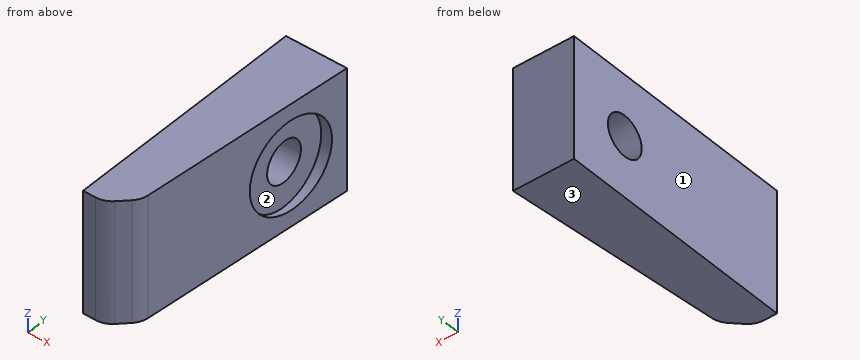
from build123d import *

# Parameters (mm, degrees)
EXTRUDE_1_DEPTH     = 30
SKETCH_3_R          = 5
CUT_EXTRUDE_2_DEPTH = 21
CUT_EXTRUDE_START   = -15
SKETCH_5_R          = 11
CUT_EXTRUDE_3_DEPTH = 3


with BuildPart() as part:
    # Эскиз1 → Бобышка-Вытянуть1 (new body)
    with BuildSketch(Plane.XY):
        with BuildLine():
            Line((0, 0), (0, -60))
            Line((0, -60), (3.117055694, -60))
            ThreePointArc((3.117055694, -60), (5.030472856, -59.619397663), (6.6525896, -58.535533906))
            Line((6.6525896, -58.535533906), (8.901294402, -56.286829104))
            ThreePointArc((8.901294402, -56.286829104), (9.897299431, -54.864386507), (10.346733987, -53.187073912))
            Line((10.346733987, -53.187073912), (15, 0))
            Line((15, 0), (0, 0))
        make_face()
    extrude(amount=EXTRUDE_1_DEPTH)

    # Эскиз3 → Вырез-Вытянуть2 (cut)
    with BuildSketch(Plane.ZY):
        with Locations((15, -15)):
            Circle(SKETCH_3_R)
    extrude(amount=-CUT_EXTRUDE_2_DEPTH, mode=Mode.SUBTRACT)

    # Эскиз5 → Вырез-Вытянуть3 (cut)
    with BuildSketch(Plane.ZY.offset(CUT_EXTRUDE_START)):
        with Locations((15, -15)):
            Circle(SKETCH_5_R)
    extrude(amount=CUT_EXTRUDE_3_DEPTH, mode=Mode.SUBTRACT)


solid = part.part
Can you work these out from the model? Positions are in its coordinate system, mm. Face numbers are marked on the shaded views. Give positions to 0.01 mm unless a question says otherwise; leave off trailing zeros. Loops run counter-clockwise (first coordinate to the right, second up) from the corner with the lowest first, then second, coordinate; pieces in that order, holes last. Notation, with made-up numbers: (32.25, 2) - (50.25, 2) arc R12 ccw to (50.25, 19) - close; hole circle Ø5 at (-14.75, -20). An arc over 180 degrees is marked (long way). One line per item, written item: value.
(1) If we section it at D-D, the plane x = 4: List the corners of the cut face in (y, z) for me.
Verdict:
outline: (-59.92, 0) - (0, 0) - (0, 30) - (-59.92, 30) - close; hole circle Ø10 at (-15, 15)
(2) If we section it at C-C, the plane z = 27.75: List the corners of the cut face in (x, y) for me, plus the area to 3 significant figures.
Verdict:
outline: (0, -60) - (3.12, -60) arc R5 ccw to (6.65, -58.54) - (8.9, -56.29) arc R5 ccw to (10.35, -53.19) - (15, 0) - (0, 0) - close
area: 730 mm^2
(3) If we mould it in two halves opening along Z, with no side actions, what happens to the marked faces 1, 2 and 3? For each: released by +Z, released by -Z, zero draft, split by the parting line, or undercut.
Verdict:
face 1: zero draft
face 2: undercut
face 3: released by -Z
(4) If we section it at B-B, the plane z = 14.75: List the corners of the cut face in (x, y) for me.
Verdict:
outline: (0, -60) - (3.12, -60) arc R5 ccw to (6.65, -58.54) - (8.9, -56.29) arc R5 ccw to (10.35, -53.19) - (12.73, -26) - (12, -26) - (12, -19.99) - (0, -19.99) - close; (0, -10.01) - (12, -10.01) - (12, -4) - (14.65, -4) - (15, 0) - (0, 0) - close
(5) If we section it at A-A, the plane y = -15: List the corners of the cut face in (x, z) for me, plus the area to 3 significant figures.
Verdict:
outline: (0, 0) - (13.69, 0) - (13.69, 4) - (12, 4) - (12, 10) - (0, 10) - close; (0, 20) - (12, 20) - (12, 26) - (13.69, 26) - (13.69, 30) - (0, 30) - close
area: 254 mm^2
(6) I need wall thicknesses on line 1 along X through (y, z) = (-23, 12); line 2 along Y through (x, z) = (14.05, 15); line 3 along Y through (x, z) = (9.25, 12.25). Which ranges of each line are inside material? Lowest first, please.
Verdict:
line 1: 0 to 12
line 2: -4 to 0
line 3: -55.9 to -19.18, -10.82 to 0
(7) I'm going to push flat-ended pins straight in: pin 1 (16 mm diameter, centred on y = -15, z = 15, fed in from -X); pin 2 (6.5 mm diameter, centred on y = -14, z = 20.5, fed in from +X); pin 3 (12 mm diameter, centred on y = -33.5, z = 9, fed in from +X); pin 4 (1.5 mm diameter, centred on x = 7.5, z = 22, fed in from -Y). Where does each tip first touch, or does it pass through?
Verdict:
pin 1: x = 0
pin 2: x = 12
pin 3: x = 12.59
pin 4: y = -58.44
